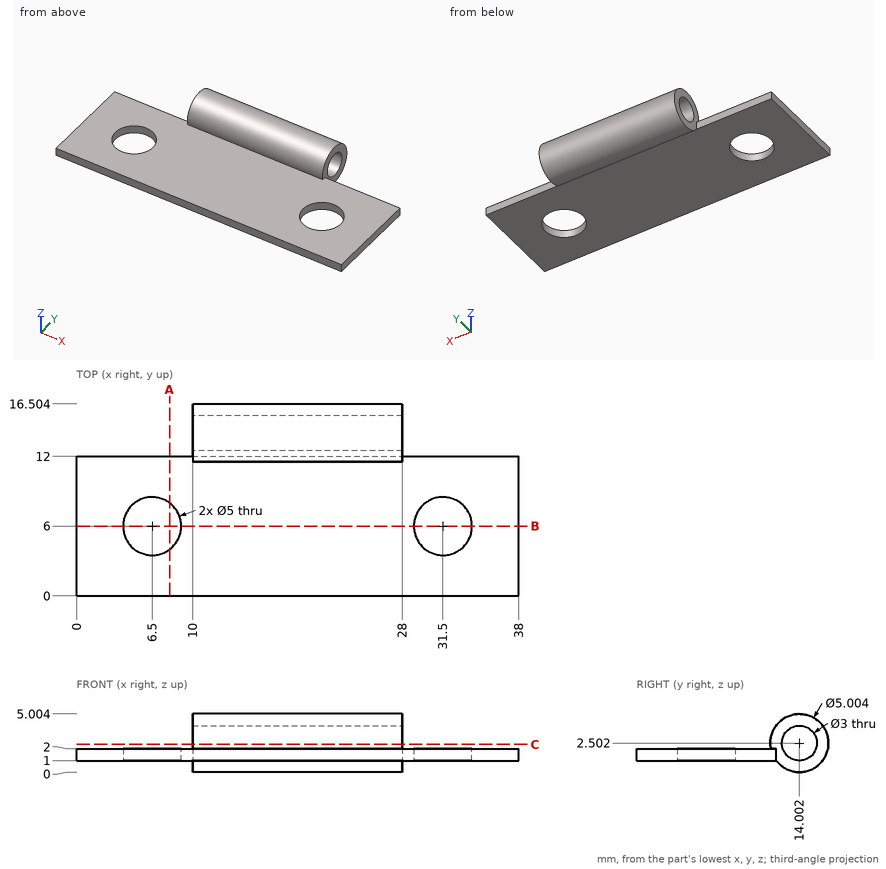
Design review of the part shown in the three views and the two pictorial views. Dimensions are in mm from the part's minimum x, y and z. Give positions to 0.01 mm unless a question says otherwise; leave off trailing zeros. Loops run counter-clockwise (first coordinate to the right, second up) from the corner with the lowest first, then second, coordinate; pieces in that order, holes last. Notation, with made-up numbers: M 65.5,30.5 L 104.5,30.5 A26 cw 104.5,68.5 Z; hole C 89,21 d10. An arc over 180 degrees is marked long. Answer as a JSON object with one key per item and string values. Group by question number.
Q1. Insertion check: P1, Ø5, axis at x = 14.5, y = 10.5, coming from the -Z side; P2, Ø9.5, axis at x = 26, y = 7, coming from the -Z side; P3, Ø3.5, axis at x = 22, y = 3, coming from the +Z side; P4, Ø4.5, axis at x = 31.5, y = 6, coming from the -Z side. Each pin has a flat end and moves straight along its axis. Give the tip position at first contact, or say it passes through.
Q2. Add section B-B on y = 6. Give the boundary of the cut face in (x, z).
Q3. Add section C-C on z = 2.4. Give the boundary of the cut face in (x, y) (1 decimal).
Q4. Add section A-A on x = 8. Give the boundary of the cut face in (y, z).
Q5. For probe 1 along Y at (x, z) = (31.5, 1.8); probe 2 along X at (y, z) = (5.5, 1.05); probe 3 along X at (y, z) = (15.5, 1), list the stretches that pass through material, from the lowest coordinate up. Write a range as [from, to].
Checked values:
{
 "1": {"P1": "z = 0.21", "P2": "z = 1", "P3": "z = 2", "P4": "through"},
 "2": {"outline": "M 0,1 L 4,1 L 4,2 L 0,2 Z; M 9,1 L 29,1 L 29,2 L 9,2 Z; M 34,1 L 38,1 L 38,2 L 34,2 Z"},
 "3": {"outline": "M 10,11.5 L 28,11.5 L 28,12.5 L 10,12.5 Z; M 10,15.5 L 28,15.5 L 28,16.5 L 10,16.5 Z"},
 "4": {"outline": "M 0,1 L 4,1 L 4,2 L 0,2 Z; M 8,1 L 12,1 L 12,2 L 8,2 Z"},
 "5": {"probe 1": "[0, 3.5], [8.5, 12]", "probe 2": "[0, 4.05], [8.95, 29.05], [33.95, 38]", "probe 3": "[10, 28]"}
}
